from build123d import *

# Parameters (mm, degrees)
SKETCH1_R           = 5
BOSS_EXTRUDE1_DEPTH = 5
SKETCH3_W           = 199.496057237
SKETCH3_H           = 5
BOSS_EXTRUDE2_DEPTH = 30
FILLET1_R           = 10
BOSS_EXTRUDE3_DEPTH = 200
FILLET2_R           = 10
SKETCH8_R           = 5
CUT_EXTRUDE1_DEPTH  = 200


with BuildPart() as part:
    # Sketch1 → Boss-Extrude1 (new body)
    with BuildSketch(Plane(origin=(0, 0, 0), x_dir=(0, 0, -1), z_dir=(1, 0, 0))):
        with BuildLine():
            Line((0, 0), (200, 0))
            Line((200, 0), (200, 190))
            ThreePointArc((200, 190), (197.071067812, 197.071067812), (190, 200))
            Line((190, 200), (10, 200))
            ThreePointArc((10, 200), (2.928932188, 197.071067812), (0, 190))
            Line((0, 190), (0, 0))
        make_face()
        with Locations((40, 40)):
            Circle(SKETCH1_R, mode=Mode.SUBTRACT)
        with Locations((40, 60)):
            Circle(SKETCH1_R, mode=Mode.SUBTRACT)
        with Locations((40, 80)):
            Circle(SKETCH1_R, mode=Mode.SUBTRACT)
        with Locations((40, 100)):
            Circle(SKETCH1_R, mode=Mode.SUBTRACT)
        with Locations((40, 120)):
            Circle(SKETCH1_R, mode=Mode.SUBTRACT)
        with Locations((40, 140)):
            Circle(SKETCH1_R, mode=Mode.SUBTRACT)
        with Locations((40, 160)):
            Circle(SKETCH1_R, mode=Mode.SUBTRACT)
        with Locations((40, 180)):
            Circle(SKETCH1_R, mode=Mode.SUBTRACT)
        with Locations((160, 180)):
            Circle(SKETCH1_R, mode=Mode.SUBTRACT)
        with Locations((160, 40)):
            Circle(SKETCH1_R, mode=Mode.SUBTRACT)
        with Locations((160, 80)):
            Circle(SKETCH1_R, mode=Mode.SUBTRACT)
        with Locations((160, 60)):
            Circle(SKETCH1_R, mode=Mode.SUBTRACT)
        with Locations((160, 100)):
            Circle(SKETCH1_R, mode=Mode.SUBTRACT)
        with Locations((160, 120)):
            Circle(SKETCH1_R, mode=Mode.SUBTRACT)
        with Locations((160, 140)):
            Circle(SKETCH1_R, mode=Mode.SUBTRACT)
        with Locations((160, 160)):
            Circle(SKETCH1_R, mode=Mode.SUBTRACT)
    extrude(amount=BOSS_EXTRUDE1_DEPTH)

    # Sketch3 → Boss-Extrude2 (add)
    with BuildSketch(Plane.ZY):
        with Locations((-99.748028619, 2.5)):
            Rectangle(SKETCH3_W, SKETCH3_H)
    extrude(amount=BOSS_EXTRUDE2_DEPTH)

    # Fillet1
    fillet1_edges = [part.edges().sort_by_distance(p)[0] for p in [
        (5, 0, -100),
    ]]
    fillet(fillet1_edges, radius=FILLET1_R)

    # Sketch7 → Boss-Extrude3 (add)
    with BuildSketch(Plane.XY):
        with BuildLine():
            Line((0, 15), (0, 5))
            Line((0, 5), (-10, 5))
            ThreePointArc((-10, 5), (-2.928932188, 7.928932188), (0, 15))
        make_face()
    extrude(amount=-BOSS_EXTRUDE3_DEPTH)

    # Fillet2
    fillet2_edges = [part.edges().sort_by_distance(p)[0] for p in [
        (-30, 2.5, -199.496057237),
        (-30, 2.5, 0),
    ]]
    fillet(fillet2_edges, radius=FILLET2_R)

    # Sketch8 → Cut-Extrude1 (cut)
    with BuildSketch(Plane(origin=(0, 5, 0), x_dir=(1, 0, 0), z_dir=(0, 1, 0))):
        with Locations(Location((-20, 169.496057237, 0), (0, 0, 270))):
            Circle(SKETCH8_R)
        with Locations(Location((-20, 29.496057237, 0), (0, 0, 270))):
            Circle(SKETCH8_R)
    extrude(amount=-CUT_EXTRUDE1_DEPTH, mode=Mode.SUBTRACT)


solid = part.part
The model under review builds one solid part; all positions refer to its coordinate system, in mm. A direction names the side the tool comes from. Coordinates: 2 decimals unless noted, no trailing zeros. Loops run counter-clockwise (first coordinate to the right, second up) from the corner with the lowest first, then second, coordinate; pieces in that order, holes last.
(1) Wall thickness on L1, parallel to X at y = 16.5, z = -49; L2, parallel to X at y = 9.5, z = -118: over which ranges is each line inside the solid? List them lowest first.
Determined:
L1: x = 0 to 5
L2: x = -1.65 to 4.99
(2) Consider section A-A, the plane y = 40. Give the boundary of the cut face in (x, z), plus the area to 3 significant figures.
Determined:
outline: (0, -200) - (5, -200) - (5, -165) - (0, -165) - close; (0, -155) - (5, -155) - (5, -45) - (0, -45) - close; (0, -35) - (5, -35) - (5, 0) - (0, 0) - close
area: 900 mm2
(3) Consider section C-C, the plane z = -27. Give the boundary of the cut face in (x, y).
Determined:
outline: (-30, 0) - (-24.33, 0) - (-24.33, 5) - (-30, 5) - close; (-15.67, 0) - (-5, 0) arc R10 ccw to (5, 10) - (5, 200) - (0, 200) - (0, 15) arc R10 cw to (-10, 5) - (-15.67, 5) - close
(4) Consider section D-D, the plane x = -27.5. Give the boundary of the cut face in (y, z).
Determined:
outline: (0, -196.11) - (5, -196.11) - (5, -3.39) - (0, -3.39) - close
(5) Draft analysis for pull direction Z (two halves, no side actions). For faces 3 (the cylindrical face through (2, 63, -36)), 4 (the cylindrical face through (2.46, 197.15, -3.01)), 5 (the flat face through (5, 106, -99)), state which applies: +Z half, -Z half, draft (parallel to the pull), parting line (faces both ways), or undercut.
Determined:
face 3: undercut
face 4: +Z half
face 5: draft
(6) Insertion check: P1, Ø16, axis at y = 40, z = -160, coming from the -X side; P2, Ø8, axis at x = -22.5, z = -136.5, coming from the +Y side; P3, Ø12, axis at x = -21.5, z = -104.5, coming from the -Y side. Each pin has a flat end and moves straight along its axis. Give the tip position at first contact, or say it passes through.
Determined:
P1: stops at x = 0
P2: stops at y = 5
P3: stops at y = 0
(7) Tool access review of faces 1 (the flat face through (0, 109, -99)), 2 (the cylindrical face through (2, 120, -155)): name each direction out of +Z, -Z, +X, -X, +Y, -Y from which nothing blocks a thin tool from reaching the whole face with its end or side.
Determined:
face 1: +Z, -Z, -X, +Y
face 2: +X, -X
(8) Consider section B-B, the plane z = -100. Give the boundary of the cut face in (x, y), plus the area to 3 significant figures.
Determined:
outline: (-30, 0) - (-5, 0) arc R10 ccw to (5, 10) - (5, 200) - (0, 200) - (0, 15) arc R10 cw to (-10, 5) - (-30, 5) - close
area: 1,150 mm2
